from build123d import *

# Parameters (mm, degrees)
F0_R     = 12.5
F1_DEPTH = 200
F3_W     = 8
F3_H     = 50
F4_DEPTH = 4
F5_R     = 3.9999
F6_R     = 0.25
F7_SIZE  = 1


# Not quite as in the source:
# - a fillet or chamfer is up to 0.001 mm smaller than in the source, because OpenCascade refuses the exact size


with BuildPart() as f1:
    # F0 (on Front) → F1 (new body)
    with BuildSketch(Plane.XZ):
        Circle(F0_R)
    extrude(amount=F1_DEPTH)

    # F3 (on offset) → F4 (cut)
    with BuildSketch(Plane.XY.offset(12.5)):
        with Locations((0, -50)):
            Rectangle(F3_W, F3_H)
    extrude(amount=-F4_DEPTH, mode=Mode.SUBTRACT)

    # F5 (radius 4 in the source; OpenCascade refuses exactly that, so slightly less here)
    f5_edges = [f1.edges().sort_by_distance(p)[0] for p in [
        (-4, -25, 10.17136),
        (4, -25, 10.17136),
        (4, -75, 10.17136),
        (-4, -75, 10.17136),
    ]]
    fillet(f5_edges, radius=F5_R)

    # F6
    f6_edges = [f1.edges().sort_by_distance(p)[0] for p in [
        (0, -25, 8.5),
        (2.828456, -26.171544, 8.5),
        (-2.828456, -26.171544, 8.5),
        (4, -50, 8.5),
        (-4, -50, 8.5),
        (2.828456, -73.828456, 8.5),
        (-2.828456, -73.828456, 8.5),
        (0, -75, 8.5),
    ]]
    fillet(f6_edges, radius=F6_R)

    # F7
    f7_edges = [f1.edges().sort_by_distance(p)[0] for p in [
        (-12.5, -200, 0),
        (-12.5, 0, 0),
    ]]
    chamfer(f7_edges, length=F7_SIZE)


solid = f1.part
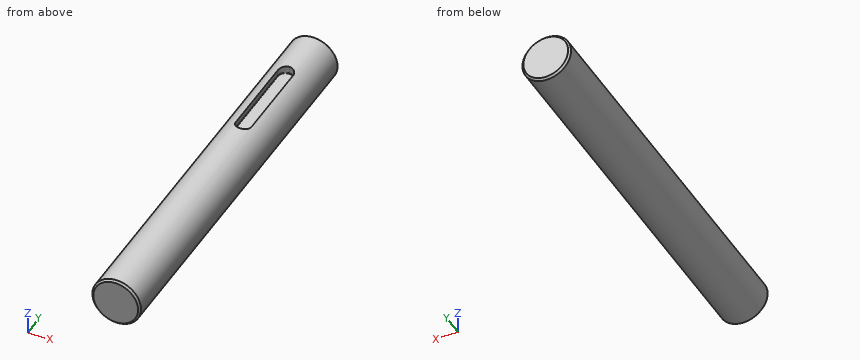
Work out the finished part from the listing and answer in its coordinate system (mm). Round coordinates to 2 decimals unless told otherwise and drop trailing zeros. Order: outer loops, then holes, each group sorted by start corner. A loop starts at its lowest first (then second) coordinate and runs counter-clockwise, first axis right, second up. Notation, with made-up numbers: M 89.25,77.25 L 104.25,77.25 A25 ccw 104.25,100.25 Z; hole C -13,-36.75 d2. An arc over 180 degrees is marked long. Put each result on its own line as item: value. Start each with the question number.
Q1. Section B-B, the plane y = -136 is taken. Write down the section's boundary in (x, z), and give its area (3 significant figures).
Q2. Straight lines are drawn through the part: L1, parallel to Z at x = 0.5, y = -155.5; L2, parallel to X at y = -162, z = -1; L3, parallel to Z at x = -1, y = -56. For each, find the intervals that lie inside material, in ascending order. Write a range as [from, to].
Q3. Flat-ended cylindrical pins translate along their axes: pin 1 (3 mm diameter, centred on x = -7, y = -107, fed in from -Z) (3 decimals); pin 2 (8 mm diameter, centred on x = -8, y = -76.5, fed in from +Z); pin 3 (4 mm diameter, centred on x = 9, y = -108, fed in from +Z). Find the tip coordinate at first contact, or state that the pin passes through.
Q4. Section A-A, the plane y = -63 is taken. Write down the section's boundary in (x, z).
Findings below:
1. outline: C 0,0 d25
1. area: 491 mm^2
2. L1: z = [-12.49, 12.49]
2. L2: x = [-12.46, 12.46]
2. L3: z = [-12.46, 8.5]
3. pin 1: stops at z = -11.225
3. pin 2: stops at z = 11.84
3. pin 3: stops at z = 10.36
4. outline: M -4,8.75 L -4,11.84 A12.5 ccw long 4,11.84 L 4,8.75 A0.25 cw 3.75,8.5 L -3.75,8.5 A0.25 cw Z
